CAD build for the part. Positions are in the model's coordinates, mm. A direction names the side the tool comes from. Give positions to 0.01 mm unless a question says otherwise; leave off trailing zeros. Order: outer loops, then holes, each group sorted by start corner. A loop starts at its lowest first (then second) coordinate and runs counter-clockwise, first axis right, second up. Notation, with made-up numbers: M 5.5,80.25 L 38.5,80.25 A21 ccw 38.5,116.25 Z; hole C -10,28.5 d10. An arc over 180 degrees is marked long. Put each result on its own line as item: value. Start each with the question number.
1) Cut at B-B (z = 12.5). Write the cut outline in (x, y).
2) Cut at A-A (y = -1). Write the cut outline in (x, z).
3) Two-plate mould, pull along Y, no slides. Class faces 5 (the face through (0, 9, 16)), 6 (the face through (-23.311, 10.483, 5.154)), 7 (the face through (-2.476, 12.232, 4.168)): released by +Y, released by -Y, zero draft, split by the parting line, or undercut.
4) Cut at C-C (z = 2.5). Write the cut outline in (x, y), and give its area (3 significant figures).
5) Tool access for faces 1 (the face through (28, 10, 5)), 2 (the face through (-20, 0, 0)), 3 (the face through (-18.665, 19.365, 4.846)), 4 (the face through (3.497, 29.722, 3.846)): list every direction of +Z, -Z, +X, -X, +Y, -Y with a clear straight run to the whole face (end or side of a thin tool).
6) Drill centre lines: line 1 (Z direction, x = 0, y = 0); line 2 (Z direction, x = -5, y = 25); line 3 (X direction, y = 24, z = -6.5). Where is each one in solid material? Low to high. Write a range as [from, to].
7) Pin check, flat tips, straight feed: pin 1 (5 mm diameter, centred on y = 17, z = 7.5, fed in from -X); pin 2 (7 mm diameter, centred on x = 19, z = 4.5, fed in from -Y); pin 3 (1.5 mm diameter, centred on y = 24.5, z = 9.5, fed in from +X); pin 4 (3 mm diameter, centred on x = 19, y = -3, fed in from -Z). Stop position of each tip, or through.
8) Cut at D-D (y = 13). Write the cut outline in (x, z), and give its area (3 significant figures).
```python
from build123d import *

# Parameters (mm, degrees)
SKETCH1_W                               = 64
SKETCH1_H                               = 32
BOSS_EXTRUDE1_DEPTH                     = 10
SKETCH4_W                               = 64
SKETCH4_H                               = 10
BOSS_EXTRUDE3_DEPTH                     = 26
BOSS_EXTRUDE4_DEPTH                     = 22
FILLET1_R                               = 3
SKETCH6_W                               = 16
SKETCH6_H                               = 9
BOSS_EXTRUDE5_DEPTH                     = 32
CBORE_FOR_M6_HEX_HEAD_BOLT1_D           = 7
CBORE_FOR_M6_HEX_HEAD_BOLT1_DEPTH       = 15
CBORE_FOR_M6_HEX_HEAD_BOLT1_CBORE_D     = 14.55
CBORE_FOR_M6_HEX_HEAD_BOLT1_CBORE_DEPTH = 4.38
CBORE_FOR_M6_HEX_HEAD_BOLT1_TIP         = 2.103012167
SKETCH12_R                              = 8
CUT_EXTRUDE1_DEPTH                      = 24
TAP_DRILL_FOR_M6X1_0_TAP1_D             = 5
TAP_DRILL_FOR_M6X1_0_TAP1_DEPTH         = 16
TAP_DRILL_FOR_M6X1_0_TAP1_TIP           = 1.502151548


with BuildPart() as part:
    # Sketch1 → Boss-Extrude1 (new body)
    with BuildSketch(Plane(origin=(0, 0, 0), x_dir=(1, 0, 0), z_dir=(0, 1, 0))):
        Rectangle(SKETCH1_W, SKETCH1_H)
    extrude(amount=BOSS_EXTRUDE1_DEPTH)

    # Sketch4 → Boss-Extrude3 (add)
    with BuildSketch(Plane(origin=(0, 10, 0), x_dir=(1, 0, 0), z_dir=(0, 1, 0))):
        with Locations((0, 11)):
            Rectangle(SKETCH4_W, SKETCH4_H)
    extrude(amount=BOSS_EXTRUDE3_DEPTH)

    # Sketch5 → Boss-Extrude4 (add)
    with BuildSketch(Plane.XY.offset(-6)):
        with BuildLine():
            Line((-15.204681896, 26.786179615), (-23.032206002, 10))
            Line((-23.032206002, 10), (21.548444147, 10))
            Line((21.548444147, 10), (13.720920041, 26.786179615))
            ThreePointArc((13.720920041, 26.786179615), (-0.741880927, 36), (-15.204681896, 26.786179615))
        make_face()
    extrude(amount=BOSS_EXTRUDE4_DEPTH)

    # Fillet1
    fillet1_edges = [part.edges().sort_by_distance(p)[0] for p in [
        (21.548444147, 10, 5),
        (-23.032206002, 10, 5),
    ]]
    fillet(fillet1_edges, radius=FILLET1_R)

    # Sketch6 → Boss-Extrude5 (add)
    with BuildSketch(Plane.XY.offset(16)):
        with Locations((0, -4.5)):
            Rectangle(SKETCH6_W, SKETCH6_H)
    extrude(amount=-BOSS_EXTRUDE5_DEPTH)

    # CBORE for M6 Hex Head Bolt1
    with Locations(Plane(origin=(0, 36, 0), x_dir=(1, 0, 0), z_dir=(0, 1, 0))):
        with Locations((0, -4)):
            CounterBoreHole(CBORE_FOR_M6_HEX_HEAD_BOLT1_D / 2, CBORE_FOR_M6_HEX_HEAD_BOLT1_CBORE_D / 2, CBORE_FOR_M6_HEX_HEAD_BOLT1_CBORE_DEPTH, depth=CBORE_FOR_M6_HEX_HEAD_BOLT1_DEPTH)
            with Locations((0, 0, -(CBORE_FOR_M6_HEX_HEAD_BOLT1_DEPTH + CBORE_FOR_M6_HEX_HEAD_BOLT1_TIP / 2))):  # 118° drill point
                Cone(0, CBORE_FOR_M6_HEX_HEAD_BOLT1_D / 2, CBORE_FOR_M6_HEX_HEAD_BOLT1_TIP, mode=Mode.SUBTRACT)

    # Sketch12 → Cut-Extrude1 (cut)
    with BuildSketch(Plane.XY.offset(16)):
        with Locations((-0.741880927, 20.042064765)):
            Circle(SKETCH12_R)
    extrude(amount=-CUT_EXTRUDE1_DEPTH, mode=Mode.SUBTRACT)

    # Tap Drill for M6x1.0 Tap1
    with Locations(Plane(origin=(0, -9, 0), x_dir=(-1, 0, 0), z_dir=(0, -1, 0))):
        with Locations((0, -8), (0, 8)):
            Hole(TAP_DRILL_FOR_M6X1_0_TAP1_D / 2, depth=TAP_DRILL_FOR_M6X1_0_TAP1_DEPTH)
            with Locations((0, 0, -(TAP_DRILL_FOR_M6X1_0_TAP1_DEPTH + TAP_DRILL_FOR_M6X1_0_TAP1_TIP / 2))):  # 118° drill point
                Cone(0, TAP_DRILL_FOR_M6X1_0_TAP1_D / 2, TAP_DRILL_FOR_M6X1_0_TAP1_TIP, mode=Mode.SUBTRACT)


solid = part.part
```
Solution:
1. outline: M -32,0 L -8,0 L -8,-9 L 8,-9 L 8,0 L 32,0 L 32,10 L 23.46,10 A3 cw 20.74,11.73 L 13.72,26.79 A15.96 ccw -15.2,26.79 L -22.22,11.73 A3 cw -24.94,10 L -32,10 Z; hole C -0.74,20.04 d16
2. outline: M -8,-16 L 8,-16 L 8,16 L -8,16 Z; hole C 0,-8 d5; hole C 0,8 d5
3. face 5: zero draft
3. face 6: released by +Y
3. face 7: undercut
4. outline: M -32,0 L -8,0 L -8,-9 L 8,-9 L 8,0 L 32,0 L 32,10 L 23.46,10 A3 cw 20.74,11.73 L 13.72,26.79 A15.96 ccw 7.12,33.93 L 7.12,31.62 L 3.16,31.62 L 3.16,27.02 A8 cw long -3.16,27.67 L -3.16,31.62 L -7.12,31.62 L -7.12,34.67 A15.96 ccw -15.2,26.79 L -22.22,11.73 A3 cw -24.94,10 L -32,10 Z
4. area: 1,310 mm²
5. face 1: +Z, +X, +Y
5. face 2: +Z, -Z, -X, -Y
5. face 3: +Z, -X, +Y
5. face 4: +Y
6. line 1: [-16, -10.5], [-5.5, 5.5], [10.5, 16]
6. line 2: [-16, -8]
6. line 3: [-32, -7.69], [6.21, 32]
7. pin 1: x = -20.93
7. pin 2: y = 0
7. pin 3: x = 15.14
7. pin 4: through
8. outline: M -32,-16 L 32,-16 L 32,-6 L 20.15,-6 L 20.15,16 L 3.05,16 L 3.05,-8 L -4.54,-8 L -4.54,16 L -21.63,16 L -21.63,-6 L -32,-6 Z
8. area: 1,380 mm²
